The listing builds one solid part. Answer for the finished solid, in the listing's coordinates (mm). Coordinates: 2 decimals unless noted, no trailing zeros. Write each loop counter-clockwise with the first axis right and the second up, starting at its lowest first coordinate (ties: lowest second). Pieces come first, ordered by that corner, then holes. Notation, with made-up numbers: M 53,16.25 L 95,16.25 A14 cw 95,22.25 Z; hole C 2,-22 d10. An arc over 180 degrees is marked long. Answer as CSV lines item,"result".
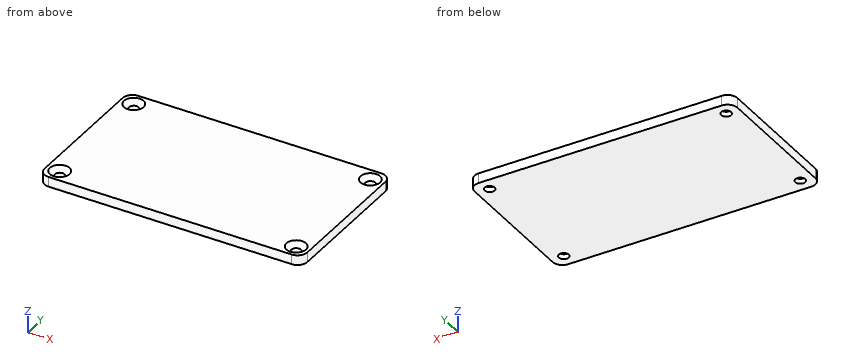
```python
from build123d import *

# Parameters (mm, degrees)
SKETCH_W     = 80
SKETCH_H     = 46
PAD_DEPTH    = 3
FILLET_R     = 3
FILLET001_R  = 3
SKETCH001_R  = 1.5
POCKET_DEPTH = 3
CHAMFER_SIZE = 1.5


with BuildPart() as part:
    # Sketch → Pad (new body)
    with BuildSketch(Plane.XY):
        with Locations((40, 23)):
            Rectangle(SKETCH_W, SKETCH_H)
    extrude(amount=PAD_DEPTH)

    # Fillet
    fillet_edges = [part.edges().sort_by_distance(p)[0] for p in [
        (80, 0, 1.5),
        (0, 0, 1.5),
    ]]
    fillet(fillet_edges, radius=FILLET_R)

    # Fillet001
    fillet001_edges = [part.edges().sort_by_distance(p)[0] for p in [
        (80, 46, 1.5),
        (0, 46, 1.5),
    ]]
    fillet(fillet001_edges, radius=FILLET001_R)

    # Sketch001 → Pocket (cut)
    with BuildSketch(Plane.XY.offset(3)):
        with Locations((4, 42)):
            Circle(SKETCH001_R)
        with Locations((4, 4)):
            Circle(SKETCH001_R)
        with Locations((76, 4)):
            Circle(SKETCH001_R)
        with Locations((76, 42)):
            Circle(SKETCH001_R)
    extrude(amount=-POCKET_DEPTH, mode=Mode.SUBTRACT)

    # Chamfer
    chamfer_edges = [part.edges().sort_by_distance(p)[0] for p in [
        (2.5, 42, 3),
        (2.5, 4, 3),
        (74.5, 4, 3),
        (74.5, 42, 3),
    ]]
    chamfer(chamfer_edges, length=CHAMFER_SIZE)


solid = part.part
```
Q1. Straight lines are drawn through the part: line 1 (Y direction, x = 4, z = 0.55); line 2 (X direction, y = 4, z = 1.6); line 3 (X direction, y = 41, z = 2.35). For each, find the intervals that lie inside material, in ascending order.
Output:
line 1,"0 to 2.5, 5.5 to 40.5, 43.5 to 46"
line 2,"0 to 2.4, 5.6 to 74.4, 77.6 to 80"
line 3,"0 to 1.87, 6.13 to 73.87, 78.13 to 80"
Q2. Find section A-A (y = 42). Give the vertices of the cut face in (x, z), and give its area (4 significant figures).
Output:
outline,"M 0,0 L 2.5,0 L 2.5,1.5 L 1,3 L 0,3 Z; M 5.5,0 L 74.5,0 L 74.5,1.5 L 73,3 L 7,3 L 5.5,1.5 Z; M 77.5,0 L 80,0 L 80,3 L 79,3 L 77.5,1.5 Z"
area,"217.5 mm2"
Q3. Find section C-C (z = 2.25). Give the vertices of the cut face in (x, y), and give its area (3 significant figures).
Output:
outline,"M 0,3 A3 ccw 3,0 L 77,0 A3 ccw 80,3 L 80,43 A3 ccw 77,46 L 3,46 A3 ccw 0,43 Z; hole C 4,4 d4.5; hole C 4,42 d4.5; hole C 76,4 d4.5; hole C 76,42 d4.5"
area,"3,610 mm2"
Q4. Find section B-B (x = 76). Give the vertices of the cut face in (y, z).
Output:
outline,"M 0,0 L 2.5,0 L 2.5,1.5 L 1,3 L 0,3 Z; M 5.5,0 L 40.5,0 L 40.5,1.5 L 39,3 L 7,3 L 5.5,1.5 Z; M 43.5,0 L 46,0 L 46,3 L 45,3 L 43.5,1.5 Z"
Q5. A flat-ended cylindrical pin translates along its axis: pin 1 Ø4 at (x, y) = (4, 42) entering from +Z. Find the tip coordinate at first contact, or state that the pin passes through.
Output:
pin 1,"z = 2"
